Design review of the part shown in the three views and the two pictorial views. Dimensions are in mm from the part's minimum x, y and z. Round coordinates to 2 decimals unless told otherwise and drop trailing zeros. Loops run counter-clockwise (first coordinate to the right, second up) from the corner with the lowest first, then second, coordinate; pieces in that order, holes last.
1. Consider section C-C on z = 2.25. State the section outline as (x, y) points, then the cut area to 3 significant figures.
2. To check wall thickness, follow line 1 along Y through (x, z) = (5.5, 6.75); line 2 along Z through (x, y) = (6, 3); line 3 along X through (y, z) = (6.5, 6.5). State the ranges of each line that lie inside material, in increasing order.
3. Clearance check with flat-ended pins moving along their axes: pin 1 Ø4 at (y, z) = (4.5, 1.5) entering from +X; pin 2 Ø4 at (x, z) = (3, 3.5) entering from -Y; pin 3 Ø4 at (y, z) = (8.5, 6) entering from -X. State where each tip first meets the part, or that it passes through.
4. Consider section A-A on y = 5.5. State the section outline as (x, z) points.
5. Draft analysis for pull direction X (two halves, no side actions). For the marked faces 1, 2 and 3, state which applies: released by +X, released by -X, zero draft, split by the parting line, or undercut.
6. Consider section D-D on z = 7.75. State the section outline as (x, y) points.
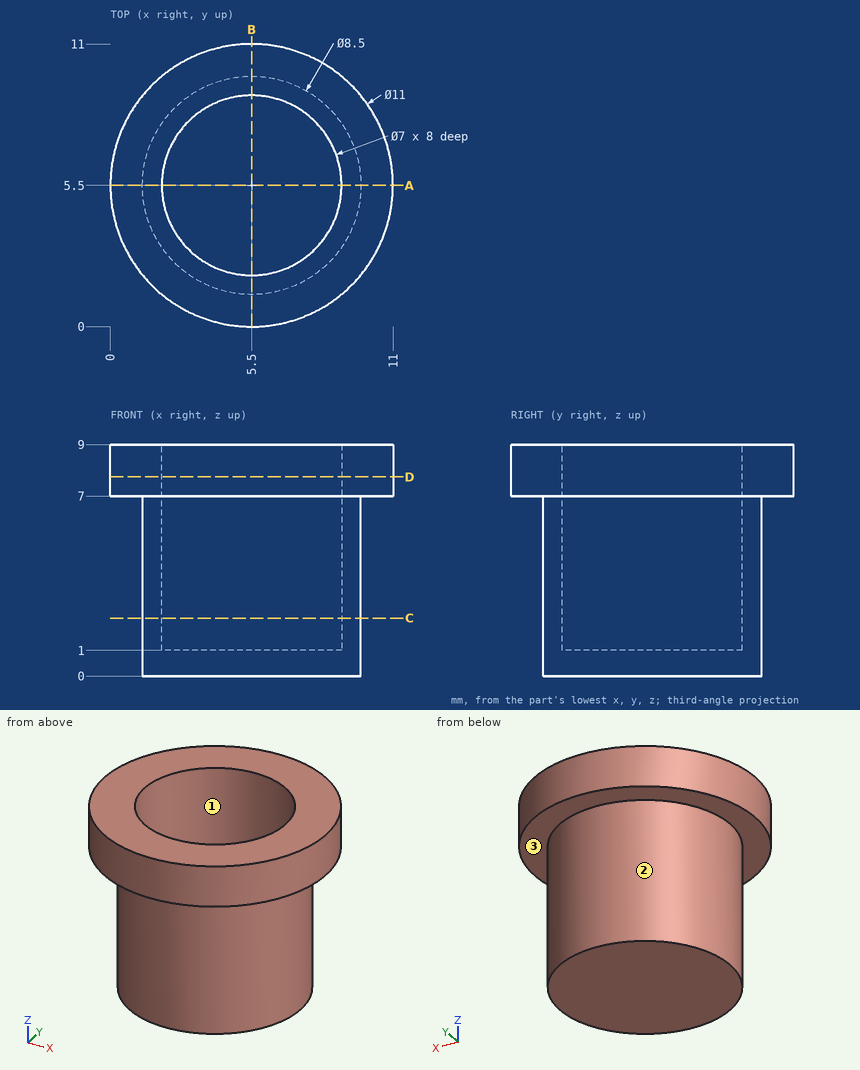
Resolved:
1. outline: circle Ø8.5 at (5.5, 5.5); hole circle Ø7 at (5.5, 5.5)
1. area: 18.3 mm2
2. line 1: y = 1.25 to 2, 9 to 9.75
2. line 2: z = 0 to 1
2. line 3: x = 1.37 to 2.15, 8.85 to 9.63
3. pin 1: stops at x = 9.75
3. pin 2: stops at y = 1.28
3. pin 3: stops at x = 0.15
4. outline: (0, 7) - (1.25, 7) - (1.25, 0) - (9.75, 0) - (9.75, 7) - (11, 7) - (11, 9) - (9, 9) - (9, 1) - (2, 1) - (2, 9) - (0, 9) - close
5. face 1: undercut
5. face 2: split by the parting line
5. face 3: zero draft
6. outline: circle Ø11 at (5.5, 5.5); hole circle Ø7 at (5.5, 5.5)
